The model under review builds one solid part; all positions refer to its coordinate system, in mm. A direction names the side the tool comes from. Round coordinates to 2 decimals unless told otherwise and drop trailing zeros. Order: outer loops, then holes, each group sorted by start corner. A loop starts at its lowest first (then second) coordinate and runs counter-clockwise, first axis right, second up. Notation, with made-up numbers: M 3,-14.5 L 10,-14.5 A19 ccw 10,17.5 Z; hole C 26,-36.75 d7. An arc over 180 degrees is marked long. Use a Markdown table: item, result. Add a question column.
1. Consider section A-A on z = 0. State the section outline as (x, y) points, then the cut area to 3 significant figures.
2. Insertion check: P1, Ø2, axis at x = 64, z = 2, coming from the -Y side. The pin has a flat end and moves straight along its axis. Give the tip position at first contact, or say it passes through.
3. To check wall thickness, follow probe 1 along X at (y, z) = (-3, -2.75); probe 2 along Y at (x, z) = (52.5, -3.25). State the ranges of each line that lie inside material, in increasing order.
4. For faces 4 (the cylindrical face through (51.631, -0.891, -4.012)), 5 (the cylindrical face through (12.04, -0.54, -2.44)), list the 3-axis set-ups (+Z, -Z, +X, -X, +Y, -Y) from which the entire face can be reached by the end or side of a thin tool; tool diameter is ignored.
5. Consider section C-C on x = 45. State the section outline as (y, z) points.
6. The part is to be moulded in two halves that separate along X. For faces 1 (the flat face through (87.25, 0, 0)), 2 (the cylindrical face through (4.563, -0.891, -4.012)), 3 (the flat face through (9, 2, -2)), say which applies: +X half, -X half, draft (parallel to the pull), parting line (faces both ways), or undercut.
Autodesk Inventor part; units mm, degrees
ref_plane "YZ Plane" through (0, 0, 0) normal (1, 0, 0) x (0, 1, 0)
ref_plane "XZ Plane" through (0, 0, 0) normal (0, 1, 0) x (-1, 0, 0)
ref_plane "XY Plane" through (0, 0, 0) normal (0, 0, 1) x (1, 0, 0)
sketch "Sketch1" plane through (0, 0, 0) normal (0, 0, 1) x (1, 0, 0)
  line L0 (0, 0) -> (0, 4.11)
  line L1 (0, 4.11) -> (9, 4.11)
  line L2 (9, 2.5) -> (9, 4.11)
  line L3 (9, 2.5) -> (15, 2.5)
  line L4 (15, 2.5) -> (15, 4.11)
  line L5 (15, 4.11) -> (87.25, 4.11)
  line L6 (0, 0) -> (87.25, 0)
  line L7 (0, 0) -> (87.25, 0)
  line L8 (87.25, 4.11) -> (87.25, 0)
  dimension "d0" = 4.11
  dimension "d1" = 9
  dimension "d3" = 6
revolve "Revolution1" add sketch "Sketch1" angle 360 about axis through (0, 0, 0) along (1, 0, 0)
properties part number "rod"
Answer block:
| question | item | result |
|---|---|---|
| 1 | outline | M 0,-4.11 L 9,-4.11 L 9,-2.5 L 15,-2.5 L 15,-4.11 L 87.25,-4.11 L 87.25,4.11 L 15,4.11 L 15,2.5 L 9,2.5 L 9,4.11 L 0,4.11 Z |
| 1 | area | 698 mm^2 |
| 2 | P1 | y = -3.99 |
| 3 | probe 1 | 0 to 9, 15 to 87.25 |
| 3 | probe 2 | -2.52 to 2.52 |
| 4 | face 4 | +X, -X |
| 4 | face 5 | none |
| 5 | outline | C 0,0 d8.22 |
| 6 | face 1 | +X half |
| 6 | face 2 | draft |
| 6 | face 3 | undercut |
